```python
from build123d import *

# Parameters (mm, degrees)
SKETCH_1_R      = 2.2
EXTRUDE_1_DEPTH = 2
SKETCH_2_R      = 5
SKETCH_2_R_2    = 2.2
EXTRUDE_3_DEPTH = 6


with BuildPart() as part:
    # 草图1 → 凸台-拉伸1 (new body)
    with BuildSketch(Plane(origin=(0, 0, 0), x_dir=(1, 0, 0), z_dir=(0, 1, 0))):
        with BuildLine():
            Line((-20, 12.5), (20, 12.5))
            ThreePointArc((20, 12.5), (23.535533906, 11.035533906), (25, 7.5))
            Line((25, 7.5), (25, -3.5))
            ThreePointArc((25, -3.5), (23.535533906, -7.035533906), (20, -8.5))
            Line((20, -8.5), (-20, -8.5))
            ThreePointArc((-20, -8.5), (-23.535533906, -7.035533906), (-25, -3.5))
            Line((-25, -3.5), (-25, 7.5))
            ThreePointArc((-25, 7.5), (-23.535533906, 11.035533906), (-20, 12.5))
        make_face()
        with Locations(Location((20, 7.5, 0), (0, 0, 270))):
            Circle(SKETCH_1_R, mode=Mode.SUBTRACT)
        with Locations(Location((-20, 7.5, 0), (0, 0, 270))):
            Circle(SKETCH_1_R, mode=Mode.SUBTRACT)
        with Locations(Location((20, -3.5, 0), (0, 0, 270))):
            Circle(SKETCH_1_R, mode=Mode.SUBTRACT)
        with Locations(Location((-20, -3.5, 0), (0, 0, 270))):
            Circle(SKETCH_1_R, mode=Mode.SUBTRACT)
    extrude(amount=EXTRUDE_1_DEPTH)

    # 草图2 → 凸台-拉伸3 (add)
    # profile 1 of 2: a face of its own
    with BuildSketch(Plane(origin=(0, 2, 0), x_dir=(1, 0, 0), z_dir=(0, 1, 0))):
        with Locations(Location((-20, -3.5, 0), (0, 0, 270))):
            Circle(SKETCH_2_R)
        with Locations(Location((-20, -3.5, 0), (0, 0, 270))):
            Circle(SKETCH_2_R_2, mode=Mode.SUBTRACT)
    # profile 2 of 2: a face of its own
    with BuildSketch(Plane(origin=(0, 2, 0), x_dir=(1, 0, 0), z_dir=(0, 1, 0))):
        with Locations(Location((20, -3.5, 0), (0, 0, 270))):
            Circle(SKETCH_2_R)
        with Locations(Location((20, -3.5, 0), (0, 0, 270))):
            Circle(SKETCH_2_R_2, mode=Mode.SUBTRACT)
    extrude(amount=EXTRUDE_3_DEPTH)


solid = part.part
```
Here's how the part is built. I have some questions about the finished solid (model axes, mm). Coordinates: 2 decimals unless noted, no trailing zeros. Loops run counter-clockwise (first coordinate to the right, second up) from the corner with the lowest first, then second, coordinate; pieces in that order, holes last. Notation, with made-up numbers: (-18, 33.25) - (34, 33.25) arc R26 cw to (34, 51.25) - close; hole circle Ø11 at (51.25, -2). An arc over 180 degrees is marked (long way). Return JSON: item names as keys, results as strings. Group by question number.
Item 1: Will these pins go through, and if not, where does the flat tip stop? P1, Ø1.5, axis at x = -13.5, z = -2, coming from the +Y side; P2, Ø3, axis at y = 5, z = -2, coming from the +X side.
Item 2: If we section it at B-B on y = 1: Write out the boundary of the cut face in (x, z), and give its area (3 significant figures).
Item 3: We'd pull the mould along X, two halves only. Please class faces 1 (the face through (0, 1, 8.5)), 2 (the face through (23.5, 0.99, -11.07)), 3 (the face through (18.05, 0.99, -6.48)): +X half, -X half, draft (parallel to the pull), parting line (faces both ways), or undercut.
Item 4: I need wall thicknesses on line 1 (X direction, y = 0.8, z = -7.5); line 2 (X direction, y = 6, z = 3.5); line 3 (Y direction, x = 11, z = 5). Which ranges of each line are inside material? Lowest first, please. Write a range as from..to.
Item 5: If we section it at C-C on x = -4.5: Write out the boundary of the cut face in (y, z), and give its area (3 significant figures).
Item 6: If we section it at A-A on y = 3.5: Write out the boundary of the cut face in (x, z), and give its area (3 significant figures).
Calculated:
{
 "1": {"P1": "stops at y = 2", "P2": "stops at x = 23"},
 "2": {"outline": "(-25, -7.5) arc R5 ccw to (-20, -12.5) - (20, -12.5) arc R5 ccw to (25, -7.5) - (25, 3.5) arc R5 ccw to (20, 8.5) - (-20, 8.5) arc R5 ccw to (-25, 3.5) - close; hole circle Ø4.4 at (-20, -7.5); hole circle Ø4.4 at (-20, 3.5); hole circle Ø4.4 at (20, -7.5); hole circle Ø4.4 at (20, 3.5)", "area": "968 mm^2"},
 "3": {"face 1": "draft", "face 2": "+X half", "face 3": "undercut"},
 "4": {"line 1": "x = -25..-22.2, -17.8..17.8, 22.2..25", "line 2": "x = -25..-22.2, -17.8..-15, 15..17.8, 22.2..25", "line 3": "y = 0..2"},
 "5": {"outline": "(0, -12.5) - (2, -12.5) - (2, 8.5) - (0, 8.5) - close", "area": "42.0 mm^2"},
 "6": {"outline": "circle Ø10 at (-20, 3.5); circle Ø10 at (20, 3.5); hole circle Ø4.4 at (-20, 3.5); hole circle Ø4.4 at (20, 3.5)", "area": "127 mm^2"}
}
